Source: CAD feature listing. Evaluate the final solid. Frame: model axes, mm. A direction names the side the tool comes from. Give positions to 0.01 mm unless a question says otherwise; leave off trailing zeros. Loops run counter-clockwise (first coordinate to the right, second up) from the corner with the lowest first, then second, coordinate; pieces in that order, holes last.
from build123d import *

# Parameters (mm, degrees)
F0_W     = 142.606944
F0_H     = 95.77182
F0_W_2   = 130.597934
F0_H_2   = 82.56191
F1_DEPTH = 76.2
F2_W     = 69.881048
F2_H     = 36.019358
F3_DEPTH = 127
F4_R     = 9.161786
F5_DEPTH = 177.8


with BuildPart() as f1:
    # F0 (on Top) → F1 (new body)
    with BuildSketch(Plane.XY):
        Rectangle(F0_W, F0_H)
        Rectangle(F0_W_2, F0_H_2, mode=Mode.SUBTRACT)
    extrude(amount=F1_DEPTH)

    # F2 (on face) → F3 (cut)
    with BuildSketch(Plane.XZ.offset(47.88591)):
        with Locations((-0.636155, 58.190321)):
            Rectangle(F2_W, F2_H)
    extrude(amount=-F3_DEPTH, mode=Mode.SUBTRACT)

    # F4 (on face) → F5 (cut)
    with BuildSketch(Plane.YZ.offset(71.303472)):
        with Locations((0, 40.680505)):
            Circle(F4_R)
    extrude(amount=-F5_DEPTH, mode=Mode.SUBTRACT)


solid = f1.part
1) Cut plane A-A (x = -5). Return loops of the section in (y, z), and give its area (3 significant figures).
Checks:
outline: (-47.89, 0) - (-41.28, 0) - (-41.28, 40.18) - (-47.89, 40.18) - close; (41.28, 0) - (47.89, 0) - (47.89, 40.18) - (41.28, 40.18) - close
area: 531 mm2
2) Ray query, probe 1 along Z at (x, y) = (68, 0); probe 2 along X at (y, z) = (-20, 23.5); probe 3 along Y at (x, z) = (3.5, 33.5). Return the intervals inside material, ascending.
Checks:
probe 1: z = 0 to 31.52, 49.84 to 76.2
probe 2: x = -71.3 to -65.3, 65.3 to 71.3
probe 3: y = -47.89 to -41.28, 41.28 to 47.89
3) Cut plane D-D (z = 34). Return loops of the section in (x, y).
Checks:
outline: (-71.3, -47.89) - (71.3, -47.89) - (71.3, -6.27) - (65.3, -6.27) - (65.3, -41.28) - (-65.3, -41.28) - (-65.3, -6.27) - (-71.3, -6.27) - close; (-71.3, 6.27) - (-65.3, 6.27) - (-65.3, 41.28) - (65.3, 41.28) - (65.3, 6.27) - (71.3, 6.27) - (71.3, 47.89) - (-71.3, 47.89) - close
4) Cut plane C-C (y = 0). Return loops of the section in (x, z).
Checks:
outline: (-71.3, 0) - (-65.3, 0) - (-65.3, 31.52) - (-71.3, 31.52) - close; (-71.3, 49.84) - (-65.3, 49.84) - (-65.3, 76.2) - (-71.3, 76.2) - close; (65.3, 0) - (71.3, 0) - (71.3, 31.52) - (65.3, 31.52) - close; (65.3, 49.84) - (71.3, 49.84) - (71.3, 76.2) - (65.3, 76.2) - close
5) Cut plane B-B (y = 34). Return loops of the section in (x, z).
Checks:
outline: (-71.3, 0) - (-65.3, 0) - (-65.3, 76.2) - (-71.3, 76.2) - close; (65.3, 0) - (71.3, 0) - (71.3, 76.2) - (65.3, 76.2) - close
6) Reachability of faces 5 (the flat face through (-1, 41.281, 29)), 6 (the flat face through (71.303, -1, 29)), 7 (the flat face through (-35.577, 45, 58)) from +Z, -Z, +X, -X, +Y, -Y: full face, straight path, thin tool, end or side. Return the list, or none.
Checks:
face 5: +Z, -Z
face 6: +Z, -Z, +X, +Y, -Y
face 7: +Z, +Y, -Y
7) Pull-direction query (Y, two-part tool) for faces 1 (the flat face through (-65.299, -1, 29)), 2 (the flat face through (65.299, -1, 29)), 3 (the flat face through (-1, 47.886, 29)), 4 (the flat face through (-1, 45, 40.181)); classes: released by +Y, released by -Y, zero draft, split by the parting line, or undercut.
Checks:
face 1: undercut
face 2: undercut
face 3: released by +Y
face 4: zero draft
8) Contact query for a flat-ended pin moving along its axis: P1, Ø7.5, axis at x = -13, y = -46, coming from the +Z side. Output: stop coordinate, or through.
Checks:
P1: stops at z = 40.18
